```python
from build123d import *

# Parameters (mm, degrees)
BOSS_EXTRUDE1_DEPTH = 2
BOSS_EXTRUDE4_DEPTH = 1.5
SKETCH4_W           = 18.96
SKETCH4_H           = 3
BOSS_EXTRUDE5_DEPTH = 3.5


with BuildPart() as part:
    # Sketch1 → Boss-Extrude1 (new body)
    with BuildSketch(Plane.XZ.offset(-30.427346286)):
        with BuildLine():
            Line((61.676013052, 15.196320566), (61.676013052, 19.156320566))
            Line((61.676013052, 19.156320566), (61.676013052, 74.528320566))
            ThreePointArc((61.676013052, 74.528320566), (56.122757624, 87.935065137), (42.716013052, 93.488320566))
            Line((42.716013052, 93.488320566), (14.268013052, 93.488320566))
            ThreePointArc((14.268013052, 93.488320566), (0.861268481, 87.935065137), (-4.691986948, 74.528320566))
            Line((-4.691986948, 74.528320566), (-4.691986948, 19.156320566))
            Line((-4.691986948, 19.156320566), (-4.691986948, 15.196320566))
            Line((-4.691986948, 15.196320566), (-4.273831516, 15.196320566))
            Line((-4.273831516, 15.196320566), (14.268013052, 15.196320566))
            Line((14.268013052, 15.196320566), (14.268013052, 20.196320566))
            Line((14.268013052, 20.196320566), (42.716013052, 20.196320566))
            Line((42.716013052, 20.196320566), (42.716013052, 15.196320566))
            Line((42.716013052, 15.196320566), (61.257857621, 15.196320566))
            Line((61.257857621, 15.196320566), (61.676013052, 15.196320566))
        make_face()
    extrude(amount=BOSS_EXTRUDE1_DEPTH)

    # Sketch3 → Boss-Extrude4 (add)
    with BuildSketch(Plane(origin=(0, 30.427346286, 0), x_dir=(1, 0, 0), z_dir=(0, 1, 0))):
        with BuildLine():
            ThreePointArc((46.676013052, -19.156320566), (45.516155906, -16.356177712), (42.716013052, -15.196320566))
            Line((42.716013052, -15.196320566), (61.676013052, -15.196320566))
            Line((61.676013052, -15.196320566), (61.676013052, -74.528320566))
            ThreePointArc((61.676013052, -74.528320566), (56.122757624, -87.935065137), (42.716013052, -93.488320566))
            Line((42.716013052, -93.488320566), (14.268013052, -93.488320566))
            ThreePointArc((14.268013052, -93.488320566), (0.861268481, -87.935065137), (-4.691986948, -74.528320566))
            Line((-4.691986948, -74.528320566), (-4.691986948, -15.196320566))
            Line((-4.691986948, -15.196320566), (14.268013052, -15.196320566))
            ThreePointArc((14.268013052, -15.196320566), (11.467870199, -16.356177712), (10.308013052, -19.156320566))
            Line((10.308013052, -19.156320566), (10.308013052, -74.528320566))
            ThreePointArc((10.308013052, -74.528320566), (11.467870199, -77.328463419), (14.268013052, -78.488320566))
            Line((14.268013052, -78.488320566), (42.716013052, -78.488320566))
            ThreePointArc((42.716013052, -78.488320566), (45.516155906, -77.328463419), (46.676013052, -74.528320566))
            Line((46.676013052, -74.528320566), (46.676013052, -19.156320566))
        make_face()
    extrude(amount=BOSS_EXTRUDE4_DEPTH)

    # Sketch4 → Boss-Extrude5 (add)
    with BuildSketch(Plane.XZ.offset(-28.427346286)):
        with Locations((4.788013052, 13.696320566)):
            Rectangle(SKETCH4_W, SKETCH4_H)
        with Locations((52.196013052, 13.696320566)):
            Rectangle(SKETCH4_W, SKETCH4_H)
    extrude(amount=-BOSS_EXTRUDE5_DEPTH)


solid = part.part
```
CAD build for the part. Positions are in the model's coordinates, mm. A direction names the side the tool comes from. Give positions to 0.01 mm unless a question says otherwise; leave off trailing zeros. Loops run counter-clockwise (first coordinate to the right, second up) from the corner with the lowest first, then second, coordinate; pieces in that order, holes last. Notation, with made-up numbers: (34, 35) -> (52, 35) arc R20 ccw to (52, 66) -> close; hole circle Ø11 at (-14, 67). An arc over 180 degrees is marked (long way). Use a Markdown table: item, result.
1. Which spindle directions (+Z, -Z, +X, -X, +Y, -Y) get a long thin tool onto all of the face, cutting with end or side? Do faces 1 (the flat face through (28, 28.427, 53)), 2 (the cylindrical face through (11.499, 31.167, 16.326)), 3 (the flat face through (42.716, 30, 15)). Say none if no direction does.
Check result:
| item | result |
|---|---|
| face 1 | +Z, -Z, +X, -X, -Y |
| face 2 | +Y |
| face 3 | -Z, +Y, -Y |
2. Wall check: L1, parallel to X at y = 30.85, z = 21.5; L2, parallel to Y at x = 19, z = 54; L3, parallel to Z at x = 44, y = 31.75. Give the ranges that are in metal, low to high. Write a range as [from, to].
Check result:
| item | result |
|---|---|
| L1 | x = [-4.69, 10.31], [46.68, 61.68] |
| L2 | y = [28.43, 30.43] |
| L3 | z = [12.2, 15.41], [78.27, 93.44] |
3. Slice it at B-B (z = 24). List the corners of the cut face in (x, y).
Check result:
| item | result |
|---|---|
| outline | (-4.69, 28.43) -> (61.68, 28.43) -> (61.68, 31.93) -> (46.68, 31.93) -> (46.68, 30.43) -> (10.31, 30.43) -> (10.31, 31.93) -> (-4.69, 31.93) -> close |
4. Slice it at A-A (y = 31.05). List the corners of the cut face in (x, z), plus the area to 3 significant figures.
Check result:
| item | result |
|---|---|
| outline | (-4.69, 12.2) -> (14.27, 12.2) -> (14.27, 15.2) arc R3.96 cw to (10.31, 19.16) -> (10.31, 74.53) arc R3.96 cw to (14.27, 78.49) -> (42.72, 78.49) arc R3.96 cw to (46.68, 74.53) -> (46.68, 19.16) arc R3.96 cw to (42.72, 15.2) -> (42.72, 12.2) -> (61.68, 12.2) -> (61.68, 74.53) arc R18.96 ccw to (42.72, 93.49) -> (14.27, 93.49) arc R18.96 ccw to (-4.69, 74.53) -> close |
| area | 2,870 mm^2 |
5. Mould opens along Z. For faces 4 (the cylindrical face through (45.485, 31.167, 77.359)), 5 (the flat face through (28, 29, 20.196)), 6 (the cylindrical face through (1.01, 30.15, 88.08)) say: pulls with the +Z half, pulls with the -Z half, needs draft (parallel to the pull), parting line crosses it, or undercut.
Check result:
| item | result |
|---|---|
| face 4 | undercut |
| face 5 | pulls with the -Z half |
| face 6 | pulls with the +Z half |
6. Slice it at C-C (x = 40). List the corners of the cut face in (y, z).
Check result:
| item | result |
|---|---|
| outline | (28.43, 20.2) -> (30.43, 20.2) -> (30.43, 78.49) -> (31.93, 78.49) -> (31.93, 93.49) -> (28.43, 93.49) -> close |
7. Flat gauge pins, fed straight in: pin 1 (0.6 mm diameter, centred on x = 30, y = 29, fed in from -Z); pin 2 (11 mm diameter, centred on x = 22.5, z = 41, fed in from +Y); pin 3 (0.8 mm diameter, centred on x = 22.5, y = 31.5, fed in from -Z). Where does each tip first touch, or does it go through?
Check result:
| item | result |
|---|---|
| pin 1 | stops at z = 20.2 |
| pin 2 | stops at y = 30.43 |
| pin 3 | stops at z = 78.49 |
8. Slice it at D-D (z = 85). List the corners of the cut face in (x, y), plus the area to 3 significant figures.
Check result:
| item | result |
|---|---|
| outline | (-1.54, 28.43) -> (58.52, 28.43) -> (58.52, 31.93) -> (-1.54, 31.93) -> close |
| area | 210 mm^2 |
